Design review of the part built by this model. Coordinates are the model's own, in mm. A direction names the side the tool comes from. Coordinates: 2 decimals unless noted, no trailing zeros. Write each loop counter-clockwise with the first axis right and the second up, starting at its lowest first coordinate (ties: lowest second). Pieces come first, ordered by that corner, then holes.
Q1. For pin 1 Ø4 at (y, z) = (-7.125, -4.95) entering from +X; pin 2 Ø8 at (y, z) = (-11.5, 8) entering from +X; pin 3 Ø3 at (y, z) = (-27.5, 4.5) entering from -X, all flat-tipped, find the tip position at first contact; note any pin that passes through.
Q2. Take a section at B-B, the plane y = -58.5. Write out the cut boundary in (x, z), plus the area to 3 significant figures.
Q3. Take a section at C-C, the plane z = 6.75. Write out the cut boundary in (x, y).
Q4. The part is to be moulded in two halves that separate along Y. For faces 1 (the cylindrical face through (8.06, -10.91, 1.23)), 2 (the flat face through (162, -74.075, -5)), 3 (the flat face through (84.35, -4.76, 7.57)), 4 (the flat face through (170, -39, -5)), say which applies: released by +Y, released by -Y, zero draft, split by the parting line, or undercut.
Q5. For L1, parallel to X at y = -67, z = 0.9; L2, parallel to Y at x = 9.25, z = 1.3; L3, parallel to X at y = -56.5, z = -6.75, list the stretches that pass through material, from the lowest coordinate up.
Q6. For faces 5 (the flat face through (85.1, -11.7, 2.5)), 6 (the flat face through (1, -39, 6)), 7 (the flat face through (2.5, -68, -5)), 8 (the flat face through (168.5, -9, -5)), list the 3-axis set-ups (+Z, -Z, +X, -X, +Y, -Y) from which the entire face can be reached by the end or side of a thin tool; tool diameter is ignored.
Q7. Take a section at A-A, the plane x = 150.5. Write out the cut boundary in (y, z) (3 decimals), plus the area to 3 significant figures.
from build123d import *

# Parameters (mm, degrees)
ESQUISSE1_W             = 171
ESQUISSE1_H             = 77
ESQUISSE1_R             = 1.5
ESQUISSE1_W_2           = 149
ESQUISSE1_H_2           = 53
BOSS_EXTRU_1_DEPTH      = 2.5
ESQUISSE2_W             = 169
ESQUISSE2_H             = 74.5
ESQUISSE2_W_2           = 160
ESQUISSE2_H_2           = 65.5
BOSS_EXTRU_2_DEPTH      = 7.5
CHANFREIN7_SIZE         = 2
CHANFREIN7_SIZE2        = 4.802328779
ESQUISSE4_W             = 142.5
ESQUISSE4_H             = 1.5
ESQUISSE4_W_2           = 1.5
ESQUISSE4_H_2           = 48.4
BOSS_EXTRU_3_DEPTH      = 10.45
ESQUISSE5_R             = 1.5
ENL_V_MAT_EXTRU_1_DEPTH = 186.554446188


with BuildPart() as part:
    # Esquisse1 → Boss.-Extru.1 (new body)
    with BuildSketch(Plane.XY):
        with Locations((85.5, -38.5)):
            Rectangle(ESQUISSE1_W, ESQUISSE1_H)
        with Locations((9.25, -10)):
            Circle(ESQUISSE1_R, mode=Mode.SUBTRACT)
        with Locations((161.75, -10)):
            Circle(ESQUISSE1_R, mode=Mode.SUBTRACT)
        with Locations((161.75, -67)):
            Circle(ESQUISSE1_R, mode=Mode.SUBTRACT)
        with Locations((9.25, -67)):
            Circle(ESQUISSE1_R, mode=Mode.SUBTRACT)
        with Locations((85.5, -38.5)):
            Rectangle(ESQUISSE1_W_2, ESQUISSE1_H_2, mode=Mode.SUBTRACT)
    extrude(amount=BOSS_EXTRU_1_DEPTH)

    # Esquisse2 → Boss.-Extru.2 (add)
    with BuildSketch(Plane.XY.offset(2.5)):
        with Locations((85.5, -38.5)):
            Rectangle(ESQUISSE2_W, ESQUISSE2_H)
        with Locations((85.5, -38.5)):
            Rectangle(ESQUISSE2_W_2, ESQUISSE2_H_2, mode=Mode.SUBTRACT)
    extrude(amount=BOSS_EXTRU_2_DEPTH)

    # Chanfrein7
    chanfrein7_edges = [part.edges().sort_by_distance(p)[0] for p in [
        (5.5, -38.5, 10),
        (85.5, -71.25, 10),
        (165.5, -38.5, 10),
        (85.5, -5.75, 10),
    ]]
    chanfrein7_side = [part.faces().sort_by_distance(p)[0] for p in [
        (85.5, -3.096923117, 10),
    ]]
    chamfer(chanfrein7_edges, length=CHANFREIN7_SIZE, length2=CHANFREIN7_SIZE2, reference=chanfrein7_side[0])

    # Esquisse4 → Boss.-Extru.3 (add)
    # profile 1 of 5: a face of its own
    with BuildSketch(Plane(origin=(0, 0, 0), x_dir=(-1, 0, 0), z_dir=(0, 0, -1))):
        with BuildLine():
            Line((-167, -2.925), (-4, -2.925))
            ThreePointArc((-4, -2.925), (-2.939339828, -3.364339828), (-2.5, -4.425))
            Line((-2.5, -4.425), (-2.5, -72.575))
            ThreePointArc((-2.5, -72.575), (-2.939339828, -73.635660172), (-4, -74.075))
            Line((-4, -74.075), (-167, -74.075))
            ThreePointArc((-167, -74.075), (-168.060660172, -73.635660172), (-168.5, -72.575))
            Line((-168.5, -72.575), (-168.5, -4.425))
            ThreePointArc((-168.5, -4.425), (-168.060660172, -3.364339828), (-167, -2.925))
        make_face()
        with BuildLine():
            Line((-167, -5.925), (-167, -71.075))
            ThreePointArc((-167, -71.075), (-166.560660172, -72.135660172), (-165.5, -72.575))
            Line((-165.5, -72.575), (-5.5, -72.575))
            ThreePointArc((-5.5, -72.575), (-4.439339828, -72.135660172), (-4, -71.075))
            Line((-4, -71.075), (-4, -5.925))
            ThreePointArc((-4, -5.925), (-4.439339828, -4.864339828), (-5.5, -4.425))
            Line((-5.5, -4.425), (-165.5, -4.425))
            ThreePointArc((-165.5, -4.425), (-166.560660172, -4.864339828), (-167, -5.925))
        make_face(mode=Mode.SUBTRACT)
    # profile 2 of 5: a face of its own
    with BuildSketch(Plane(origin=(0, 0, 0), x_dir=(-1, 0, 0), z_dir=(0, 0, -1))):
        with Locations((-85.5, -2.175)):
            Rectangle(ESQUISSE4_W, ESQUISSE4_H)
    # profile 3 of 5: a face of its own
    with BuildSketch(Plane(origin=(0, 0, 0), x_dir=(-1, 0, 0), z_dir=(0, 0, -1))):
        with Locations((-169.25, -38.5)):
            Rectangle(ESQUISSE4_W_2, ESQUISSE4_H_2)
    # profile 4 of 5: a face of its own
    with BuildSketch(Plane(origin=(0, 0, 0), x_dir=(-1, 0, 0), z_dir=(0, 0, -1))):
        with Locations((-85.5, -74.825)):
            Rectangle(ESQUISSE4_W, ESQUISSE4_H)
    # profile 5 of 5: a face of its own
    with BuildSketch(Plane(origin=(0, 0, 0), x_dir=(-1, 0, 0), z_dir=(0, 0, -1))):
        with Locations((-1.75, -38.5)):
            Rectangle(ESQUISSE4_W_2, ESQUISSE4_H_2)
    extrude(amount=BOSS_EXTRU_3_DEPTH)

    # Esquisse5 → Enlèv. mat.-Extru.1 (cut, through all)
    with BuildSketch(Plane(origin=(168.5, 0, 0), x_dir=(0, 0, -1), z_dir=(1, 0, 0))):
        with Locations(Location((4.95, -7.125, 0), (0, 0, 53.130102354))):
            Circle(ESQUISSE5_R)
        with Locations((4.95, -69.875)):
            Circle(ESQUISSE5_R)
    extrude(amount=-ENL_V_MAT_EXTRU_1_DEPTH, mode=Mode.SUBTRACT)


solid = part.part
Responses:
1. pin 1: stops at x = 168.5
1. pin 2: stops at x = 170
1. pin 3: stops at x = 1
2. outline: (0, 0) - (1, 0) - (1, -10.45) - (4, -10.45) - (4, 0) - (11, 0) - (11, 2.5) - (5.5, 2.5) - (5.5, 5.2) - (3.5, 10) - (1, 10) - (1, 2.5) - (0, 2.5) - close; (160, 0) - (167, 0) - (167, -10.45) - (170, -10.45) - (170, 0) - (171, 0) - (171, 2.5) - (170, 2.5) - (170, 10) - (167.5, 10) - (165.5, 5.2) - (165.5, 2.5) - (160, 2.5) - close
2. area: 176 mm2
3. outline: (1, -75.75) - (170, -75.75) - (170, -1.25) - (1, -1.25) - close; hole (4.85, -71.9) - (166.15, -71.9) - (166.15, -5.1) - (4.85, -5.1) - close
4. face 1: undercut
4. face 2: released by -Y
4. face 3: undercut
4. face 4: zero draft
5. L1: x = 0 to 7.75, 10.75 to 160.25, 163.25 to 171
5. L2: y = -77 to -68.5, -65.5 to -11.5, -8.5 to 0
5. L3: x = 1 to 4, 167 to 170
6. face 5: +Z
6. face 6: +Z, -X, +Y, -Y
6. face 7: -Z, -X, -Y
6. face 8: -Z, +X, +Y
7. outline: (-77, 0) - (-75.575, 0) - (-75.575, -10.45) - (-72.575, -10.45) - (-72.575, 0) - (-65, 0) - (-65, 2.5) - (-71.25, 2.5) - (-71.25, 5.198) - (-73.25, 10) - (-75.75, 10) - (-75.75, 2.5) - (-77, 2.5) - close; (-12, 0) - (-4.425, 0) - (-4.425, -10.45) - (-1.425, -10.45) - (-1.425, 0) - (0, 0) - (0, 2.5) - (-1.25, 2.5) - (-1.25, 10) - (-3.75, 10) - (-5.75, 5.198) - (-5.75, 2.5) - (-12, 2.5) - close
7. area: 181 mm2
